Solid Edge part; units mm, degrees
sketch "Sketch1" plane through (0, 0, 0) normal (0, 0, 1) x (1, 0, 0)
  line L0 (0, 0) -> (0, -50)
  line L1 (0, 0) -> (0, 50)
  arc A0 (0, 50) -> (0, -50) centre (0, 0) cw
extrude "Protrusion1" add sketch "Sketch1" along normal blind 25
extrude "Protrusion2" [suppressed]
sketch "Sketch2" plane through (0, 0, 0) normal (0, -1, 0) x (1, 0, 0)
  arc A0 (25, 30) -> (-15, 70) centre (25, 70) cw
  line L0 (-15, 70) -> (-45, 70)
  arc A1 (25, 0) -> (-45, 70) centre (25, 70) cw
  line L1 (25, 0) -> (25, 30)
extrude "ExtrudedProtrusion_4" add sketch "Sketch2" along normal mid plane 30
sketch "Sketch3" plane through (25, 0, 25) normal (0, 0, 1) x (1, 0, 0)
  line L0 (22.697, 15) -> (4.697, 15)
  line L1 (4.697, 15) -> (4.697, -15)
  line L2 (4.697, -15) -> (22.697, -15)
extrude "ExtrudedCutout_1" cut sketch "Sketch3" against normal blind 5 material side at (38.697, 14.95, 25)
sketch "Sketch4" plane through (0, 0, 12.5) normal (-1, 0, 0) x (0, -1, 0)
  line L0 (5, 33.5) -> (5, 57.5)
  line L1 (-5, 33.5) -> (5, 33.5)
  line L2 (-5, 57.5) -> (-5, 33.5)
extrude "ExtrudedCutout_2" cut sketch "Sketch4" along normal blind 66.0062 material side at (0, -4.95, 58)
Model file for the job. Use its own axes, mm. A direction names the side the tool comes from. Give positions to 0.01 mm unless a question says otherwise; leave off trailing zeros. Loops run counter-clockwise (first coordinate to the right, second up) from the corner with the lowest first, then second, coordinate; pieces in that order, holes last. Notation, with made-up numbers: M 77.25,50.5 L 133.25,50.5 A9 ccw 133.25,59.5 Z; hole C -0.5,-19.5 d9. An arc over 180 degrees is marked long. Use one line per item in the form item = value.
Item 1: Slice it at A-A on y = 0. List the corners of the cut face in (x, z), and give its area (3 significant figures).
Filled in:
outline = M -40.76,46 A70 ccw 0,4.62 L 0,0 L 50,0 L 50,20 L 29.7,20 L 29.7,25 L 25,25 L 25,30 A40 cw -7,46 Z
area = 2,410 mm^2
Item 2: Flat gauge pins, fed straight in: pin 1 Ø8 at (y, z) = (-37, 10) entering from +X; pin 2 Ø10 at (x, y) = (10.5, 17.5) entering from +Z; pin 3 Ø6 at (x, y) = (38, -28.5) entering from +Z. Where does each tip first touch, or does it go through?
Filled in:
pin_1 = 37.56
pin_2 = 34.71
pin_3 = 25
Item 3: Slice it at D-D on x = 34. List the corners of the cut face in (y, z).
Filled in:
outline = M -36.66,0 L 36.66,0 L 36.66,25 L 15,25 L 15,20 L -15,20 L -15,25 L -36.66,25 Z
Item 4: Slice it at B-B on x = 2. List the corners of the cut face in (y, z), and give its area (3 significant figures).
Filled in:
outline = M -49.96,0 L 49.96,0 L 49.96,25 L 15,25 L 15,37.27 L -15,37.27 L -15,25 L -49.96,25 Z
area = 2,870 mm^2
Item 5: Drill centre lines: L1, parallel to Z at x = 25, y = -43; L2, parallel to Y at x = -17, z = 35.5; L3, parallel to Y at x = 37.5, z = 24. Where is each one in solid material? Low to high.
Filled in:
L1 = 0 to 25
L2 = -15 to 15
L3 = -33.07 to -15, 15 to 33.07
Item 6: Which spindle directions (+Z, -Z, +X, -X, +Y, -Y) get a long thin tool onto all of the face, cutting with end or side? Do faces 5 (the flat face through (-24, 0, 46)), 6 (the cylindrical face through (-32.326, 0.21, 29.829)), 7 (the flat face through (40, 0, 20)). Say none if no direction does.
Filled in:
face_5 = +Z, +X, -X
face_6 = -Z, -X, +Y, -Y
face_7 = +Z, +X
Item 7: Slice it at C-C on z = 28. List the corners of the cut face in (x, y).
Filled in:
outline = M -31,-15 L 25,-15 L 25,15 L -31,15 Z
Item 8: Two-plate mould, pull along Y, no slides. Class faces 1 (the flat face through (25, 0, 27)), 2 (the flat face through (29.697, 0, 23)), 3 (the flat face through (-30, -5, 58)), 4 (the cylindrical face through (49.988, 1.099, 12.325)): released by +Y, released by -Y, zero draft, split by the parting line, or undercut.
Filled in:
face_1 = zero draft
face_2 = undercut
face_3 = undercut
face_4 = split by the parting line
